from build123d import *

# Parameters (mm, degrees)
BOSS_EXTRUDE1_DEPTH = 4
FILLET1_R           = 3
SKETCH2_R           = 1.75
BOSS_EXTRUDE2_DEPTH = 2
BOSS_EXTRUDE3_START = -1
SKETCH3_R           = 2
BOSS_EXTRUDE3_DEPTH = 1


with BuildPart() as part:
    # Sketch1 → Boss-Extrude1 (new body)
    with BuildSketch(Plane(origin=(0, 0, 0), x_dir=(1, 0, 0), z_dir=(0, 1, 0))):
        with BuildLine():
            Line((-12.5, 9.463815789), (12.5, 9.463815789))
            add(Edge.make_bspline(
                [(12.5, 9.463815789), (7.5, -27.869517544), (-7.5, -27.869517544), (-12.5, 9.463815789)],
                knots=[0, 0, 0, 0, 1, 1, 1, 1], degree=3))
        make_face()
    extrude(amount=BOSS_EXTRUDE1_DEPTH)

    # Fillet1
    fillet1_edges = [part.edges().sort_by_distance(p)[0] for p in [
        (0, 4, -9.463815789),
        (0.023803991, 4, 18.536113697),
    ]]
    fillet(fillet1_edges, radius=FILLET1_R)

    # Sketch2 → Boss-Extrude2 (add)
    with BuildSketch(Plane.XZ):
        with Locations((0, 6.536184211)):
            Circle(SKETCH2_R)
    extrude(amount=BOSS_EXTRUDE2_DEPTH)

    # Sketch3 → Boss-Extrude3 (add)
    with BuildSketch(Plane.XZ.offset(2).offset(BOSS_EXTRUDE3_START)):
        with Locations((0, 6.536184211)):
            Circle(SKETCH3_R)
    extrude(amount=BOSS_EXTRUDE3_DEPTH)


solid = part.part
Check sheet for the modelled part. Datum: model origin and axes. Units: mm. A direction names the side the tool comes from. Round coordinates to 2 decimals unless told otherwise and drop trailing zeros.
1. Scan lines: probe 1 along Y at (x, z) = (-3.75, -1); probe 2 along Z at (x, y) = (0.25, 0.5); probe 3 along X at (y, z) = (1.5, 4). Record each from-to range of solid material in increasing order.
2. Gauge pin test, flat end, axial feed: pin 1 Ø2 at (x, y) = (-8.5, 1) entering from +Z. Record the tip position at first contact, or that the pin passes through.
3. Mould release check, pull along Y, two halves, no side actions. Record for faces 1 (the flat face through (-0.2, 0.5, -9.464)), 2 (the cylindrical face through (-0.379, -0.493, 4.828)), 3 (the flat face through (0, 4, 2)): released by +Y, released by -Y, zero draft, split by the parting line, or undercut.
4. Set-up check for faces 4 (the cylindrical face through (-0.26, -1.49, 8.52)), 5 (the flat face through (0, -2, 7)): record each of +Z, -Z, +X, -X, +Y, -Y from which the full face is reachable in a straight line by a thin tool's end or side.
Recorded:
1. probe 1: y = 0 to 4
1. probe 2: z = -9.46 to 18.53
1. probe 3: x = -9.83 to 9.83
2. pin 1: stops at z = 10.85
3. face 1: zero draft
3. face 2: undercut
3. face 3: released by +Y
4. face 4: -Y
4. face 5: +Z, -Z, +X, -X, -Y
